Part model, mm, in its own coordinate system. A direction names the side the tool comes from. Coordinates: 2 decimals unless noted, no trailing zeros. Loops run counter-clockwise (first coordinate to the right, second up) from the corner with the lowest first, then second, coordinate; pieces in that order, holes last. Notation, with made-up numbers: (-23.5, 49.25) - (9.5, 49.25) arc R34 ccw to (9.5, 79.25) - close; hole circle Ø2 at (21, -1). An arc over 180 degrees is marked (long way). Use a Markdown table: item, result. Add a question column.
1) Drop flat-ended pins along their axis: P1, Ø3.5, axis at x = 27.1, y = -10.26, coming from the +Z side; P2, Ø0.6, axis at y = 9.5, z = 1, coming from the +X side; P3, Ø6, axis at x = 27.1, y = 19.74, coming from the -Z side; P4, Ø3, axis at y = 21.5, z = 1, coming from the +X side. Give the stop position or say it passes through.
2) Pull direction Y, two halves, no side cores. Call faces 1 (the face through (-5.67, 12.31, 3.94)), 2 (the face through (0.99, -13.04, 3.94)), 3 (the face through (34.347, 4, 5)), 4 (the face through (25.02, 18.88, 4.96)): +Y half, -Y half, draft (parallel to the pull), parting line (faces both ways), or undercut.
3) Band-saw the part on B-B (z = 7). Give the cut face in (x, y), plus the area to 3 significant figures.
4) Tool access for faces 5 (the face through (2, 12, 0)), 6 (the face through (19.347, 4, 1)), 7 (the face through (-8.62, 2.74, 3.94)): list every direction of +Z, -Z, +X, -X, +Y, -Y with a clear straight run to the whole face (end or side of a thin tool).
5) Band-saw the part on C-C (y = 15). Give the cut face in (x, z), plus the area to 3 significant figures.
6) Band-saw the part on A-A (x = -14.5). Give the cut face in (y, z).
7) Probe probe 1 along Z at (x, y) = (30.5, -10); probe 2 along X at (y, z) = (-8.5, 7.25); probe 3 along Y at (x, z) = (-1, 7.25). List the from-to ranges inside material, lowest first. Write a range as [from, to].
8) Band-saw the part on D-D (x = -4). Give the cut face in (y, z), plus the area to 3 significant figures.
from build123d import *

# Parameters (mm, degrees)
EXTRUSION1_DEPTH = 8
ESQUISSE5_W      = 17.091778577
ESQUISSE5_H      = 76.980294062
EXTRUSION3_DEPTH = 2
ESQUISSE6_R      = 2.25
EXTRUSION4_DEPTH = 7


with BuildPart() as part:
    # Esquisse1 → Extrusion1 (new body)
    with BuildSketch(Plane.XY):
        with BuildLine():
            Line((34.346799903, -30.256527517), (34.346799903, 39.743472483))
            Line((34.346799903, 39.743472483), (19.346799903, 34.283918969))
            ThreePointArc((19.346799903, 34.283918969), (16.761888626, 33.052257025), (14.45811141, 31.351854722))
            ThreePointArc((14.45811141, 31.351854722), (3.093427207, 25.046605726), (-9.882286187, 24.309670273))
            ThreePointArc((-9.882286187, 24.309670273), (-16.583574554, 23.095028583), (-20.952955866, 17.870937546))
            Line((-20.952955866, 17.870937546), (10.05690062, 6.584272816))
            ThreePointArc((10.05690062, 6.584272816), (13.045263007, 0.175708995), (6.636699186, -2.812653392))
            Line((6.636699186, -2.812653392), (-24.3170743, 8.453598795))
            ThreePointArc((-24.3170743, 8.453598795), (-23.983225962, 0.807214745), (-18.340349525, -4.363528846))
            ThreePointArc((-18.340349525, -4.363528846), (1.25940449, -13.185565307), (19.346799903, -24.796974003))
            Line((19.346799903, -24.796974003), (34.346799903, -30.256527517))
        make_face()
    extrude(amount=EXTRUSION1_DEPTH)

    # Esquisse5 → Extrusion3 (cut)
    with BuildSketch(Plane(origin=(0, 0, 0), x_dir=(-1, 0, 0), z_dir=(0, 0, -1))):
        with Locations((-27.892689192, 3.666825014)):
            Rectangle(ESQUISSE5_W, ESQUISSE5_H)
    extrude(amount=-EXTRUSION3_DEPTH, mode=Mode.SUBTRACT)

    # Esquisse6 → Extrusion4 (cut, through all)
    with BuildSketch(Plane(origin=(0, 0, 2), x_dir=(-1, 0, 0), z_dir=(0, 0, -1))):
        with Locations((-27.096799903, 19.743472483)):
            Circle(ESQUISSE6_R)
        with Locations((-27.096799903, -10.256527517)):
            Circle(ESQUISSE6_R)
    extrude(amount=-EXTRUSION4_DEPTH, mode=Mode.SUBTRACT)


solid = part.part
Answer block:
| question | item | result |
|---|---|---|
| 1 | P1 | through |
| 1 | P2 | x = 19.35 |
| 1 | P3 | z = 2 |
| 1 | P4 | x = 34.35 |
| 2 | face 1 | undercut |
| 2 | face 2 | -Y half |
| 2 | face 3 | draft |
| 2 | face 4 | undercut |
| 3 | outline | (-24.32, 8.45) arc R10 ccw to (-18.34, -4.36) arc R145.6 cw to (19.35, -24.8) - (34.35, -30.26) - (34.35, 39.74) - (19.35, 34.28) arc R15 ccw to (14.46, 31.35) arc R29.14 cw to (-9.88, 24.31) arc R10 ccw to (-20.95, 17.87) - (10.06, 6.58) arc R5 cw to (6.64, -2.81) - close; hole circle Ø4.5 at (27.1, -10.26); hole circle Ø4.5 at (27.1, 19.74) |
| 3 | area | 2,180 mm2 |
| 4 | face 5 | -Z, +X, -X, +Y, -Y |
| 4 | face 6 | -Z, +X, +Y, -Y |
| 4 | face 7 | +Z, -Z |
| 5 | outline | (-13.07, 0) - (19.35, 0) - (19.35, 2) - (34.35, 2) - (34.35, 8) - (-13.07, 8) - close |
| 5 | area | 349 mm2 |
| 6 | outline | (-5.82, 0) - (4.88, 0) - (4.88, 8) - (-5.82, 8) - close; (15.52, 0) - (24.01, 0) - (24.01, 8) - (15.52, 8) - close |
| 7 | probe 1 | [2, 8] |
| 7 | probe 2 | [-8.18, 25.69], [28.5, 34.35] |
| 7 | probe 3 | [-11.99, -0.03], [10.61, 24.18] |
| 8 | outline | (-10.47, 0) - (1.06, 0) - (1.06, 8) - (-10.47, 8) - close; (11.7, 0) - (23.92, 0) - (23.92, 8) - (11.7, 8) - close |
| 8 | area | 190 mm2 |
